```python
from build123d import *

# Parameters (mm, degrees)
SKETCH_1_W          = 74
SKETCH_1_H          = 14.8
EXTRUDE_1_DEPTH     = 14.8
SKETCH_2_W          = 10
SKETCH_2_H          = 10
CUT_EXTRUDE_1_DEPTH = 65
SKETCH_3_R          = 3.9
EXTRUDE_2_DEPTH     = 10
SKETCH_4_R          = 3.9
EXTRUDE_3_DEPTH     = 25
CHAMFER_1_SIZE      = 5
CUT_EXTRUDE_2_DEPTH = 6
SKETCH_8_R          = 1.5
CUT_EXTRUDE_4_DEPTH = 50.8
SKETCH_9_W          = 7.8
SKETCH_9_H          = 7.8
SKETCH_9_R          = 1.5
EXTRUDE_4_DEPTH     = 3.1
SKETCH_10_W         = 7.8
SKETCH_10_H         = 7.8
EXTRUDE_5_DEPTH     = 3.1
SKETCH_11_W         = 10
SKETCH_11_H         = 3
CUT_EXTRUDE_5_DEPTH = 10


with BuildPart() as part:
    # Эскиз1 → Бобышка-Вытянуть1 (new body)
    with BuildSketch(Plane(origin=(0, 0, 0), x_dir=(0, 0, -1), z_dir=(1, 0, 0))):
        Rectangle(SKETCH_1_W, SKETCH_1_H)
    extrude(amount=EXTRUDE_1_DEPTH)

    # Эскиз2 → Вырез-Вытянуть1 (cut)
    with BuildSketch(Plane(origin=(0, 0, -37), x_dir=(-1, 0, 0), z_dir=(0, 0, -1))):
        with Locations((-7.4, 0)):
            Rectangle(SKETCH_2_W, SKETCH_2_H)
    extrude(amount=-CUT_EXTRUDE_1_DEPTH, mode=Mode.SUBTRACT)

    # Эскиз3 → Бобышка-Вытянуть2 (add)
    with BuildSketch(Plane(origin=(14.8, 0, 0), x_dir=(0, 0, -1), z_dir=(1, 0, 0))):
        with Locations(Location((-33.1, 0, 0), (0, 0, 180))):  # turned: the seam where the file's is
            Circle(SKETCH_3_R)
    extrude(amount=EXTRUDE_2_DEPTH)

    # Эскиз4 → Бобышка-Вытянуть3 (add)
    with BuildSketch(Plane.ZY):
        with Locations((33.1, 0)):
            Circle(SKETCH_4_R)
    extrude(amount=EXTRUDE_3_DEPTH)

    # Фаска1
    chamfer_1_edges = [part.edges().sort_by_distance(p)[0] for p in [
        (7.4, 7.4, 37),
        (7.4, -7.4, 37),
    ]]
    chamfer(chamfer_1_edges, length=CHAMFER_1_SIZE)

    # Эскиз5 → Вырез-Вытянуть2 (cut)
    with BuildSketch(Plane.ZY.offset(25)):
        Polygon((30.011815854, 2.11733764), (33.920911448, 3.653232048), (36.188184146, -2.11733764), (32.279088552, -3.653232048), align=None)
    extrude(amount=-CUT_EXTRUDE_2_DEPTH, mode=Mode.SUBTRACT)

    # Эскиз8 → Вырез-Вытянуть4 (cut, through all)
    with BuildSketch(Plane(origin=(24.8, 0, 0), x_dir=(0, 0, -1), z_dir=(1, 0, 0))):
        with Locations((-33.1, 0)):
            Circle(SKETCH_8_R)
    extrude(amount=-CUT_EXTRUDE_4_DEPTH, mode=Mode.SUBTRACT)

    # Эскиз9 → Бобышка-Вытянуть4 (add)
    with BuildSketch(Plane.ZY):
        with Locations((33.1, 0)):
            Rectangle(SKETCH_9_W, SKETCH_9_H)
        with Locations(Location((33.1, 0, 0), (0, 0, 180))):  # turned: the seam where the file's is
            Circle(SKETCH_9_R, mode=Mode.SUBTRACT)
    extrude(amount=EXTRUDE_4_DEPTH)

    # Эскиз10 → Бобышка-Вытянуть5 (add)
    with BuildSketch(Plane(origin=(14.8, 0, 0), x_dir=(0, 0, -1), z_dir=(1, 0, 0))):
        with Locations((-33.1, 0)):
            Rectangle(SKETCH_10_W, SKETCH_10_H)
    extrude(amount=EXTRUDE_5_DEPTH)

    # Эскиз11 → Вырез-Вытянуть5 (cut, through all)
    with BuildSketch(Plane(origin=(0, 0, 28), x_dir=(-1, 0, 0), z_dir=(0, 0, -1))):
        with Locations((-7.4, 3.5)):
            Rectangle(SKETCH_11_W, SKETCH_11_H)
    extrude(amount=-CUT_EXTRUDE_5_DEPTH, mode=Mode.SUBTRACT)


solid = part.part
```
Input: part model. Units: mm. Frame: model coordinates. A direction names the side the tool comes from. Give positions to 0.01 mm unless a question says otherwise; leave off trailing zeros. Order: outer loops, then holes, each group sorted by start corner. A loop starts at its lowest first (then second) coordinate and runs counter-clockwise, first axis right, second up.
1. Material intervals for L1, parallel to X at y = -3, z = 11; L2, parallel to Y at x = 6, z = 7.5; L3, parallel to Y at x = 23, z = 33, sorted ascending.
Derived:
L1: x = 0 to 2.4, 12.4 to 14.8
L2: y = -7.4 to -5, 5 to 7.4
L3: y = -3.9 to -1.5, 1.5 to 3.9
2. Reachability of faces 5 (the flat face through (17.9, -3, 30)), 6 (the flat face through (-22.04, 0.81, 35.04)), 7 (the flat face through (-2, -3.9, 33)), 8 (the flat face through (17.9, 3, 30)), 9 (the flat face through (0, -3.5, 36.6)) from +Z, -Z, +X, -X, +Y, -Y: full face, straight path, thin tool, end or side. Return the list, or none.
Derived:
face 5: -Z, +X, -Y
face 6: -X
face 7: +Z, -Z, -X, -Y
face 8: -Z, +X, +Y
face 9: +Z, -Y
3. Section C-C on x = 17. Return the cut outline in (y, z).
Derived:
outline: (-3.9, 29.2) - (3.9, 29.2) - (3.9, 37) - (-3.9, 37) - close
4. Section B-B on z = 22. Return the cut outline in (x, y).
Derived:
outline: (0, -7.4) - (14.8, -7.4) - (14.8, 7.4) - (0, 7.4) - close; hole (2.4, -5) - (12.4, -5) - (12.4, 5) - (2.4, 5) - close
5. Mould query, pull axis Z, two halves, no side actions, for faces 1 (the flat face through (7, -5, -5)), 2 (the flat face through (-22.04, -0.81, 31.16)), 3 (the flat face through (-22.042, 2.875, 31.939)), 4 (the flat face through (2, 0, -37)). Classes: released by +Z, released by -Z, zero draft, split by the parting line, or undercut.
Derived:
face 1: zero draft
face 2: undercut
face 3: undercut
face 4: released by -Z
6. Pin query (flat end, axial travel): pin 1 (3.5 mm diameter, centred on x = 16, y = -0.5, fed in from -Z); pin 2 (1.5 mm diameter, centred on y = -2, z = -16.5, fed in from -X); pin 3 (2.5 mm diameter, centred on x = -1, z = 33.5, fed in from +Y); pin 4 (0.9 mm diameter, centred on y = 0, z = 33.5, fed in from -X). Return the tip coordinate at first contact, or that it passes through.
Derived:
pin 1: stops at z = -37
pin 2: stops at x = 0
pin 3: stops at y = 6.65
pin 4: stops at x = 14.8
7. Section A-A on x = 9.5. Return the cut outline in (y, z), and give its area (3 significant figures).
Derived:
outline: (-7.4, -37) - (-5, -37) - (-5, 28) - (2, 28) - (2, 37) - (-2.4, 37) - (-7.4, 32) - close; (5, -37) - (7.4, -37) - (7.4, 32) - (5, 34.4) - close; hole circle Ø3 at (0, 33.1)
area: 390 mm2
